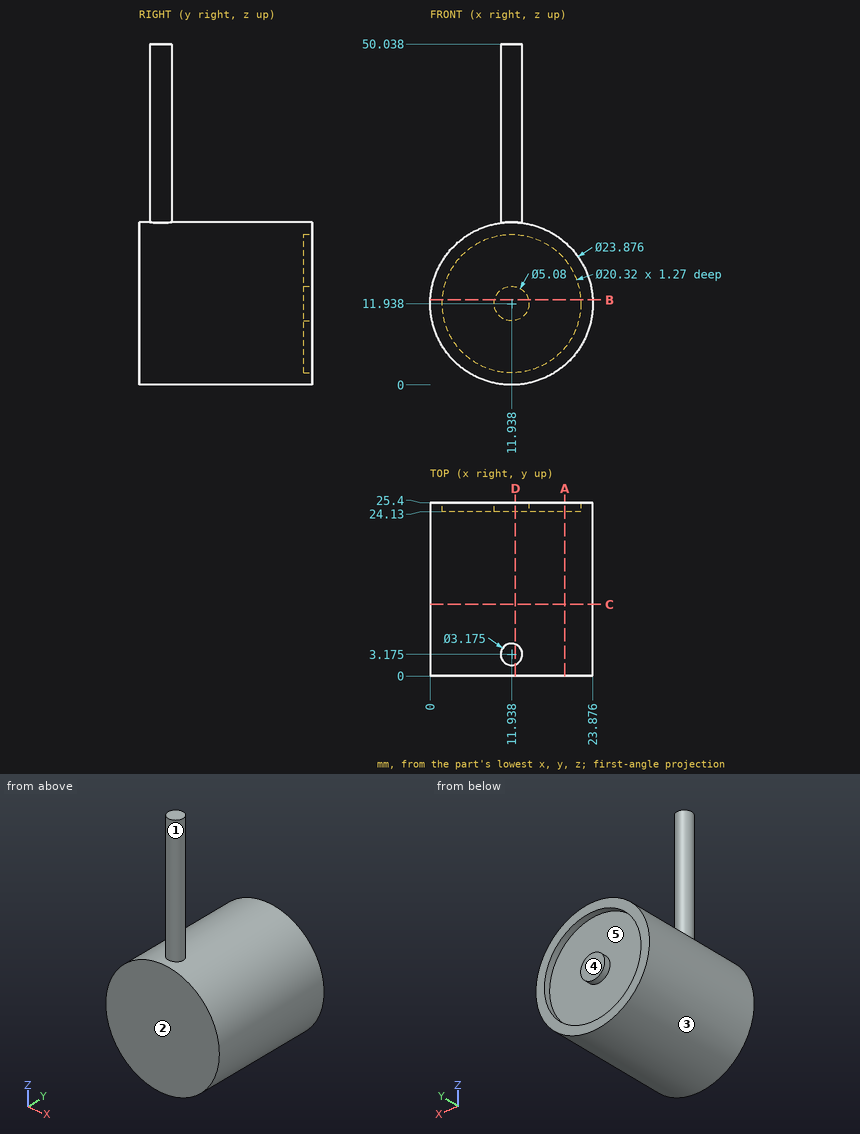
Part print with two shaded views. Sizes in mm from the minimum x, y, z corner. A direction names the side the tool comes from. Coordinates: 2 decimals unless noted, no trailing zeros. Write each loop counter-clockwise with the first axis right and the second up, starting at its lowest first coordinate (ties: lowest second). Pieces come first, ordered by that corner, then holes.
(1) Cut at B-B on z = 12.5. List the corners of the cut face in (x, y), and give its area (3 significant figures).
(2) 3-axis set-ups, long thin cutter, end or side, ignore diameter. For the marked faces 1 and 2: which of +Z, -Z, +X, -X, +Y, -Y reach the whole face in a straight line?
(3) Cut at A-A on x = 19.75. List the corners of the cut face in (y, z).
(4) Mould opens along X. For the marked faces 3, 4 and 5 say: pulls with the +X half, pulls with the -X half, needs draft (parallel to the pull), parting line crosses it, or undercut.
(5) Cut at D-D on x = 12.5. List the corners of the cut face in (y, z), and give its area (3 significant figures).
(6) Cut at C-C on y = 10.5. List the corners of the cut face in (x, z), and give its area (3 significant figures).
(7) Drill centre lines: line 1 (Y direction, x = 17.25, z = 18); line 2 (X direction, y = 4.25, z = 34); line 3 (Z direction, x = 13.75, y = 21.25). Where is each one in solid material? Low to high.
(8) Pin check, flat tips, straight feed: pin 1 Ø8 at (x, z) = (19, 34) entering from +Y; pin 2 Ø8 at (x, y) = (7, 3.5) entering from -Z; pin 3 Ø1 at (y, z) = (4.5, 20) entering from -X; pin 4 Ø5 at (y, z) = (17, 20) entering from +X. Stop position of each tip, or through.
Working result:
1. outline: (0.01, 0) - (23.86, 0) - (23.86, 25.4) - (22.08, 25.4) - (22.08, 24.13) - (14.42, 24.13) - (14.42, 25.4) - (9.46, 25.4) - (9.46, 24.13) - (1.79, 24.13) - (1.79, 25.4) - (0.01, 25.4) - close
1. area: 586 mm2
2. face 1: +Z
2. face 2: +Z, -Z, +X, -X, -Y
3. outline: (0, 2.91) - (25.4, 2.91) - (25.4, 5.44) - (24.13, 5.44) - (24.13, 18.43) - (25.4, 18.43) - (25.4, 20.97) - (0, 20.97) - close
4. face 3: parting line crosses it
4. face 4: needs draft
4. face 5: undercut
5. outline: (0, 0.01) - (25.4, 0.01) - (25.4, 1.79) - (24.13, 1.79) - (24.13, 9.46) - (25.4, 9.46) - (25.4, 14.42) - (24.13, 14.42) - (24.13, 22.08) - (25.4, 22.08) - (25.4, 23.86) - (4.66, 23.86) - (4.66, 50.04) - (1.69, 50.04) - (1.69, 23.86) - (0, 23.86) - close
5. area: 664 mm2
6. outline: circle Ø23.88 at (11.94, 11.94)
6. area: 448 mm2
7. line 1: y = 0 to 24.13
7. line 2: x = 10.77 to 13.11
7. line 3: z = 0.14 to 23.74
8. pin 1: passes through
8. pin 2: stops at z = 0.04
8. pin 3: stops at x = 2.7
8. pin 4: stops at x = 22.5
